Geometry: final body of the model. Coordinates: model frame, mm. Round coordinates to 2 decimals unless told otherwise and drop trailing zeros. Order: outer loops, then holes, each group sorted by start corner. A loop starts at its lowest first (then second) coordinate and runs counter-clockwise, first axis right, second up. Notation, with made-up numbers: M -26,9 L 11,9 A8 cw 11,17 Z; hole C 56,-28 d3. An arc over 180 degrees is marked long. Put each result on its own line as item: value. Start each with the question number.
1) Material intervals for probe 1 along X at (y, z) = (5.25, 0.6); probe 2 along X at (y, z) = (8.5, -1.85); probe 3 along Y at (x, z) = (-12, -0.5), sorted ascending. Write a range as [from, to].
2) First-contact query: P1, Ø12, axis at x = -18, y = -0.5, coming from the -Z side (3 decimals); P2, Ø2, axis at x = -6.5, z = -0.5, coming from the +Y side. Flat tips, straight axial feed; report the tip coordinate or a pass-through.
3) Section C-C, the plane x = 36. Return loops of the section in (y, z).
4) Section B-B, the plane z = 0.25. Count the separate pieces of the cut face and the enclosed holes in it, then the cut area to 3 significant figures.
5) Section D-D, the plane x = -8. Return loops of the section in (y, z).
6) Section A-A, the plane x = 13.5. Return loops of the section in (y, z).
from build123d import *

# Parameters (mm, degrees)
SKETCH005_R   = 2
SKETCH005_R_2 = 2.65
PAD_DEPTH     = 4
FILLET_R      = 15
FILLET001_R   = 1
FILLET002_R   = 1


with BuildPart() as part:
    # Sketch005 → Pad (new body)
    with BuildSketch(Plane.XY.offset(-3)):
        Polygon((-50.5, -19), (42, -19), (42, 10), (9, 10), (9, -10), (-31, -10), (-31, 10), (-50.5, 10), align=None)
        with Locations((-35.5, 5)):
            Circle(SKETCH005_R, mode=Mode.SUBTRACT)
        with Locations((-35.5, -5)):
            Circle(SKETCH005_R, mode=Mode.SUBTRACT)
        with Locations((13.5, 5)):
            Circle(SKETCH005_R, mode=Mode.SUBTRACT)
        with Locations((13.5, -5)):
            Circle(SKETCH005_R, mode=Mode.SUBTRACT)
        with Locations((-44.5, -8)):
            Circle(SKETCH005_R_2, mode=Mode.SUBTRACT)
        with Locations((-44.5, 5)):
            Circle(SKETCH005_R_2, mode=Mode.SUBTRACT)
        with Locations((22.5, -5)):
            Circle(SKETCH005_R_2, mode=Mode.SUBTRACT)
        with Locations((36, 2.5)):
            Circle(SKETCH005_R_2, mode=Mode.SUBTRACT)
    extrude(amount=PAD_DEPTH)

    # Fillet
    fillet_edges = [part.edges().sort_by_distance(p)[0] for p in [
        (-50.5, -19, -1),
        (42, -19, -1),
    ]]
    fillet(fillet_edges, radius=FILLET_R)

    # Fillet001
    fillet001_edges = [part.edges().sort_by_distance(p)[0] for p in [
        (42, 10, -1),
        (9, 10, -1),
        (-31, 10, -1),
        (-50.5, 10, -1),
    ]]
    fillet(fillet001_edges, radius=FILLET001_R)

    # Fillet002
    fillet002_edges = [part.edges().sort_by_distance(p)[0] for p in [
        (-31, -10, -1),
        (9, -10, -1),
    ]]
    fillet(fillet002_edges, radius=FILLET002_R)


solid = part.part
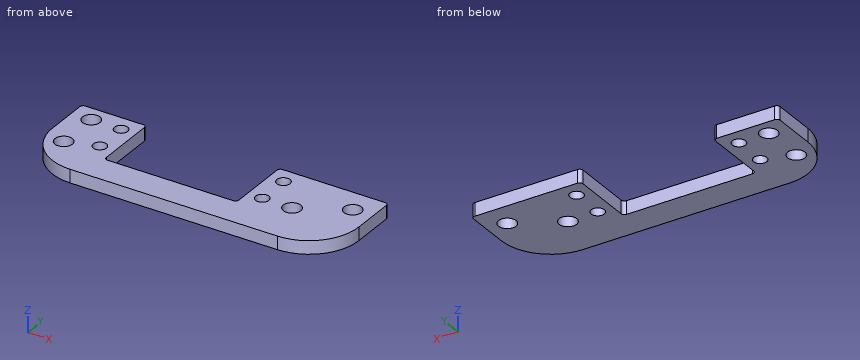
Result sheet:
1. probe 1: x = [-50.5, -47.14], [-41.86, -37.48], [-33.52, -31], [9, 11.52], [15.48, 42]
1. probe 2: x = [-50.5, -31], [9, 42]
1. probe 3: y = [-19, -10]
2. P1: passes through
2. P2: stops at y = -10
3. outline: M -16,-3 L -0.15,-3 L -0.15,1 L -16,1 Z; M 5.15,-3 L 10,-3 L 10,1 L 5.15,1 Z
4. separate pieces: 1
4. enclosed holes: 8
4. area: 1,650 mm2
5. outline: M -19,-3 L -10,-3 L -10,1 L -19,1 Z
6. outline: M -19,-3 L -7,-3 L -7,1 L -19,1 Z; M -3,-3 L 3,-3 L 3,1 L -3,1 Z; M 7,-3 L 10,-3 L 10,1 L 7,1 Z
